Design review of the part built by this model. Coordinates are the model's own, in mm. Face numbers are marked on the shaded views. A direction names the side the tool comes from. Round coordinates to 2 decimals unless told otherwise and drop trailing zeros. Loops run counter-clockwise (first coordinate to the right, second up) from the corner with the lowest first, then second, coordinate; pieces in that order, holes last. Notation, with made-up numbers: M 8,31 L 20,31 A23 cw 20,49 Z; hole C -27.75,88 d4. An arc over 180 degrees is marked long. Answer as CSV lines item,"result". Start each with the question number.
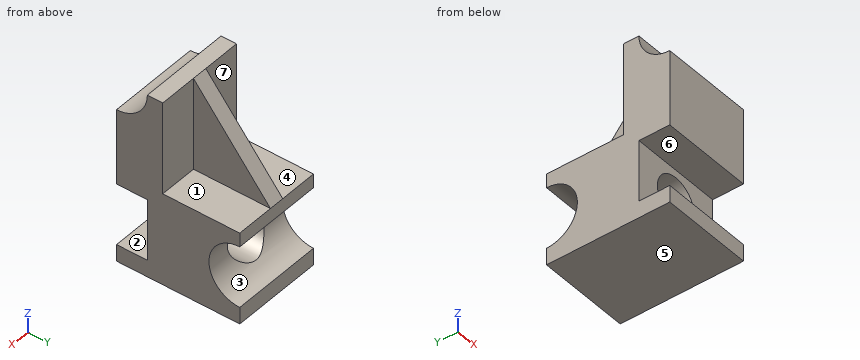
Autodesk Inventor part; units mm, degrees
ref_plane "YZ Plane" through (0, 0, 0) normal (1, 0, 0) x (0, 1, 0)
ref_plane "XZ Plane" through (0, 0, 0) normal (0, 1, 0) x (-1, 0, 0)
ref_plane "XY Plane" through (0, 0, 0) normal (0, 0, 1) x (1, 0, 0)
sketch "Эскиз1" plane through (0, 0, 0) normal (1, 0, 0) x (0, 1, 0)
  line L0 (0, -30.9291) -> (80, -30.9291)
  line L1 (80, 29.0709) -> (30, 29.0709)
  line L2 (30, 29.0709) -> (30, 89.0709)
  line L3 (30, 89.0709) -> (20, 89.0709)
  line L4 (80, 29.0709) -> (30, 89.0709)
  arc A0 (0, 69.0709) -> (20, 89.0709) centre (0, 89.0709) ccw
  arc A1 (80, 20) -> (80, -20) centre (80, 0) ccw
  line L5 (0, 20) -> (20, 20)
  line L6 (20, 20) -> (20, -20)
  line L7 (20, -20) -> (0, -20)
  line L8 (0, -20) -> (0, -30.9291)
  line L9 (80, -30.9291) -> (80, -20)
  line L10 (80, 20) -> (80, 29.0709)
  line L11 (0, 69.0709) -> (0, 20)
  point P0 (0, 0)
extrude "Выдавливание1" add sketch "Эскиз1" along normal mid plane 60 contours L8 L7 L6 L5 L11 A0 L3 L2 L1 L10 A1 L9 L0
extrude "Выдавливание2" add sketch "Эскиз1" along normal mid plane 10 contours L1 L2 L4
sketch "Эскиз3" plane through (0, 0, 0) normal (0, 1, 0) x (-1, 0, 0)
  circle A0 centre (0, 0) radius 15
  dimension "d12" = 30
extrude "Выдавливание3" cut sketch "Эскиз3" along normal blind 100
properties part number "Корпус"
Item 1: Consider section A-A, the plane x = 0. Write out the cut boundary in (y, z), then the cut area to 3 significant figures.
Item 2: To check wall thickness, follow line 1 (X direction, y = 36, z = 0); line 2 (Y direction, x = 9, z = 59); line 3 (Z direction, x = -12, y = 49.5). State the ranges of each line that lie inside material, in increasing order.
Item 3: Consider section C-C, the plane y = 53. Write out the cut boundary in (x, z).
Item 4: Insertion check: pin 1 Ø6 at (y, z) = (52.5, 53) entering from +X; pin 2 Ø1.5 at (x, z) = (5, -17.5) entering from +Y; pin 3 Ø12.5 at (x, y) = (16.5, 64.5) entering from +Z. Each pin has a flat end and moves straight along its axis. Give the tip position at first contact, or say it passes through.
Item 5: Tool access review of the marked faces 1, 2, 3 and 4: name each direction out of +Z, -Z, +X, -X, +Y, -Y from which nothing blocks a thin tool from reaching the whole face with its end or side.
Item 6: The part is to be moulded in two halves that separate along Z. For the marked faces 5, 6 and 7, say which applies: +Z half, -Z half, draft (parallel to the pull), parting line (faces both ways), or undercut.
Item 7: Consider section D-D, the plane y = 72. Write out the cut boundary in (x, z), then the cut area to 3 significant figures.
Item 8: Consider section B-B, the plane z = 0. Write out the cut boundary in (x, y).
Found:
1,outline,"M 0,-30.93 L 80,-30.93 L 80,-20 A20 cw 66.77,-15 L 20,-15 L 20,-20 L 0,-20 Z; M 0,20 L 20,20 L 20,15 L 66.77,15 A20 cw 80,20 L 80,29.07 L 30,89.07 L 20,89.07 A20 cw 0,69.07 Z"
1,area,"5,100 mm^2"
2,line 1,"x = -30 to -15, 15 to 30"
2,line 2,"y = 0 to 30"
2,line 3,"z = -30.93 to -9, 9 to 29.07"
3,outline,"M -30,-30.93 L 30,-30.93 L 30,29.07 L 5,29.07 L 5,61.47 L -5,61.47 L -5,29.07 L -30,29.07 Z; hole C 0,0 d30"
4,pin 1,"stops at x = 5"
4,pin 2,"stops at y = 71.82"
4,pin 3,"stops at z = 29.07"
5,face 1,"+Z, +X, +Y"
5,face 2,"+X, -X, -Y"
5,face 3,"+X, -X, +Y"
5,face 4,"+Z, -X, +Y"
6,face 5,"-Z half"
6,face 6,"undercut"
6,face 7,"draft"
7,outline,"M -30,-30.93 L 30,-30.93 L 30,-18.33 L -30,-18.33 Z; M -30,18.33 L 30,18.33 L 30,29.07 L 5,29.07 L 5,38.67 L -5,38.67 L -5,29.07 L -30,29.07 Z"
7,area,"1,500 mm^2"
8,outline,"M -30,20 L -15,20 L -15,60 L -30,60 Z; M 15,20 L 30,20 L 30,60 L 15,60 Z"
